Design review of the part built by this model. Coordinates are the model's own, in mm. A direction names the side the tool comes from. Coordinates: 2 decimals unless noted, no trailing zeros. Loops run counter-clockwise (first coordinate to the right, second up) from the corner with the lowest first, then second, coordinate; pieces in that order, holes last. Notation, with made-up numbers: (-17, 88.25) -> (7, 88.25) arc R25 ccw to (7, 125.25) -> close; hole circle Ø1 at (86, 33). An arc over 180 degrees is marked (long way). Answer as a JSON object with one key per item and string values.
Autodesk Inventor part; units mm, degrees
ref_plane "YZ Plane" through (0, 0, 0) normal (1, 0, 0) x (0, 1, 0)
ref_plane "XZ Plane" through (0, 0, 0) normal (0, 1, 0) x (-1, 0, 0)
ref_plane "XY Plane" through (0, 0, 0) normal (0, 0, 1) x (1, 0, 0)
sketch "TopSketch" plane through (0, 0, 0) normal (0, 1, 0) x (-1, 0, 0)
  line L0 (-39.75, -16.5) -> (39.75, -16.5)
  line L1 (39.75, -16.5) -> (39.75, 16.5)
  line L2 (39.75, 16.5) -> (-39.75, 16.5)
  line L3 (-39.75, 16.5) -> (-39.75, -16.5)
  line L4 (-39.75, -16.5) -> (39.75, 16.5) construction
  line L5 (39.75, -16.5) -> (-39.75, 16.5) construction
  point P0 (0, 0)
  dimension "EncoderSupportOutside_Length" = 33
  dimension "EncoderSupportOutside_Width" = 79.5
extrude "Top" add sketch "TopSketch" along normal blind 10
sketch "SideSketch" plane through (0, 0, 0) normal (0, -1, 0) x (1, 0, 0)
  line L0 (39.75, -16.5) -> (-39.75, -16.5)
  line L1 (39.75, 16.5) -> (39.75, -16.5)
  line L2 (-39.75, 16.5) -> (39.75, 16.5)
  line L3 (-39.75, -16.5) -> (-39.75, 16.5)
  line L4 (-29.75, 16.5) -> (-29.75, -16.5)
  line L5 (29.75, 16.5) -> (29.75, -16.5)
  line L6 (0, 0) -> (0, 21.6169) construction
  dimension "d4" = 10
extrude "Side" add sketch "SideSketch" along normal blind 51.5 contours L0 L5 L2 L1 | L0 L3 L2 L4
sketch "CableHoleSketch" plane through (0, 10, 0) normal (0, 1, 0) x (1, 0, 0)
  line L0 (-39.75, -16.5) -> (39.75, -16.5)
  line L1 (39.75, -16.5) -> (39.75, 16.5)
  line L2 (0, 0) -> (0, 14.5107) construction
  circle A0 centre (0, 18.5) radius 4.75
  dimension "d7" = 9.5
  dimension "d8" = 35
extrude "CableHole" cut sketch "CableHoleSketch" against normal up to next
sketch "InnerFasteningHoleSketch" plane through (0, 10, 0) normal (0, 1, 0) x (1, 0, 0)
  line L0 (39.75, 16.5) -> (-39.75, 16.5)
  line L1 (39.75, 16.5) -> (-39.75, 16.5)
  circle A0 centre (-24.25, 11.5) radius 2
  line L2 (0, 0) -> (39.099, 0) construction
  line L3 (0, 0) -> (0, 35.9734) construction
  circle A1 centre (-24.25, -11.5) radius 2
  circle A2 centre (24.25, 11.5) radius 2
  circle A3 centre (24.25, -11.5) radius 2
  dimension "d11" = 4
  dimension "d12" = 5
  dimension "d13" = 24.25
extrude "InnerFasteningHole" cut sketch "InnerFasteningHoleSketch" against normal up to next
sketch "OuterFasteningHoleSketch" plane through (0, 10, 0) normal (0, 1, 0) x (1, 0, 0)
  line L0 (39.75, 16.5) -> (-39.75, 16.5)
  line L1 (-39.75, 16.5) -> (-39.75, -16.5)
  line L2 (39.75, 16.5) -> (-39.75, 16.5)
  circle A0 centre (-34.75, 11.5) radius 1.75
  line L3 (0, 0) -> (36.9685, 0) construction
  line L4 (0, 0) -> (0, 24.5431) construction
  circle A1 centre (34.75, 11.5) radius 1.75
  circle A2 centre (-34.75, -11.5) radius 1.75
  circle A3 centre (34.75, -11.5) radius 1.75
  dimension "d16" = 3.5
  dimension "d17" = 5
  dimension "d18" = 5
extrude "OuterFasteningHole" cut sketch "OuterFasteningHoleSketch" against normal up to next
sketch "CoilSpringHoleSketch" plane through (0, 0, 0) normal (0, -1, 0) x (1, 0, 0)
  circle A0 centre (24.25, -11.5) radius 2
  circle A1 centre (-24.25, -11.5) radius 2
  circle A2 centre (-24.25, 11.5) radius 2
  circle A3 centre (24.25, 11.5) radius 2
  line L0 (29.75, -16.5) -> (-29.75, -16.5)
  circle A4 centre (-24.25, 11.5) radius 3
  line L1 (0, 0) -> (0, 23.1959) construction
  line L2 (0, 0) -> (47.7515, 0) construction
  circle A5 centre (24.25, 11.5) radius 3
  circle A6 centre (-24.25, -11.5) radius 3
  circle A7 centre (24.25, -11.5) radius 3
  point P0 (-4.3084, -16.5)
  dimension "d21" = 6
extrude "CoilSpringHole" cut sketch "CoilSpringHoleSketch" against normal blind 5
sketch "Sketch7" plane through (0, 0, 0) normal (0, -1, 0) x (1, 0, 0)
  circle A0 centre (-24.25, 11.5) radius 3
  arc A1 (4.3084, -16.5) -> (-4.3084, -16.5) centre (0, -18.5) ccw
  line L0 (-29.75, 16.5) -> (-29.75, -16.5)
  line L1 (-29.75, 5.5) -> (-23, 5.5)
  line L2 (-23, 5.5) -> (-23, -5.5)
  line L3 (-23, -5.5) -> (-29.75, -5.5)
  line L4 (-29.75, -5.5) -> (-29.75, 5.5)
  line L5 (0, 0) -> (50.1862, 0) construction
  line L6 (0, 0) -> (0, -18.5) construction
  line L7 (29.75, 5.5) -> (23, 5.5)
  line L8 (23, 5.5) -> (23, -5.5)
  line L9 (23, -5.5) -> (29.75, -5.5)
  line L10 (29.75, -5.5) -> (29.75, 5.5)
  circle A2 centre (-24.25, 11.5) radius 3 construction
  dimension "d25" = 3
  dimension "d26" = 23
extrude "Extrusion7" add sketch "Sketch7" along normal up to surface (51.5 mm away) contours L1 L2 L3 L0 | L10 L9 L8 L7
fillet "Fillet" radius 2 8 edges at (-29.75, -25.75, 5.5) (-23, -25.75, 5.5) (-23, -25.75, -5.5) (-29.75, -25.75, -5.5) (29.75, -25.75, 5.5) (23, -25.75, 5.5) (23, -25.75, -5.5) (29.75, -25.75, -5.5)
fillet "Fillet" radius 2 10 edges at (39.75, -20.75, -16.5) (-39.75, -20.75, -16.5) (22.0292, 10, -16.5) (0, 10, -13.75) (-22.0292, 10, -16.5) (39.75, 10, 0) (0, 10, 16.5) (-39.75, 10, 0) (-39.75, -20.75, 16.5) (39.75, -20.75, 16.5)
equation "\"EncoderSupportOutside_Length\" = EncoderSupportInside_Length"
equation "\"EncoderSupportOutside_Width\" = EncoderSupportInside_Width + 2 * EncoderSupportOutside_Thickness + 2 * EncoderSupportOutside_MecanicalSpace"
equation "\"d2\" = EncoderSupportOutside_Thickness"
equation "\"d4\" = EncoderSupportOutside_Thickness"
equation "\"d5\" = EncoderSupportInside_Height + EncoderSupport_Space"
equation "\"d7\" = Encoder_CableBase_Diameter + EncoderSupport_PlasticShrinkingMargin"
equation "\"d8\" = Encoder_CableBase_DistanceToTop + EncoderSupportInside_Front_Thickness"
equation "\"d9\" = EncoderSupportOutside_Thickness"
equation "\"d11\" = EncoderSupport_PlasticShrinkingMargin + EncoderSupport_FixingHole_Diameter + EncoderSupportOutside_MecanicalSpace"
equation "\"d12\" = EncoderSupport_FixingnHole_Margin"
equation "\"d14\" = EncoderSupportOutside_Thickness"
equation "\"d16\" = EncoderSupport_FixingHole_Diameter + EncoderSupport_PlasticShrinkingMargin"
equation "\"d17\" = EncoderSupport_FixingnHole_Margin"
equation "\"d18\" = EncoderSupport_FixingnHole_Margin"
equation "\"d19\" = EncoderSupportOutside_Thickness"
equation "\"d21\" = EncoderSupport_CoilSpringHole_Diameter"
equation "\"d25\" = EncoderSupportInside_Hollow_Margin + EncoderSupportOutside_MecanicalSpace"
equation "\"d29\" = EncoderSupport_Fillet_Size"
equation "\"EncoderSupportOutside_Thickness\" = 10"
equation "\"EncoderSupportOutside_MecanicalSpace\" = 0.5"
equation "\"EncoderSupport_Space\" = 5"
properties part number "EncoderSupportOutside" material "Polyethylene, High Density"
1) Add section C-C, the plane x = 34.75. Give the boundary of the cut face in (y, z), and give its area (3 significant figures).
Completed:
{"outline": "(-51.5, -16.5) -> (8, -16.5) arc R2 ccw to (10, -14.5) -> (10, -13.25) -> (-51.5, -13.25) -> close; (-51.5, -9.75) -> (10, -9.75) -> (10, 9.75) -> (-51.5, 9.75) -> close; (-51.5, 13.25) -> (10, 13.25) -> (10, 14.5) arc R2 ccw to (8, 16.5) -> (-51.5, 16.5) -> close", "area": "1,600 mm²"}
2) The part is to be moulded in two halves that separate along Z. For faces 4 (the cylindrical face through (-27.247, 2.465, 11.632)), 5 (the flat face through (-33, -51.5, 0)), 6 (the flat face through (26, -25, -5.5)), say which applies: pulls with the +Z half, pulls with the -Z half, needs draft (parallel to the pull), parting line crosses it, or undercut.
Completed:
{"face 4": "undercut", "face 5": "needs draft", "face 6": "pulls with the -Z half"}
3) Clearance check with flat-ended pins moving along their axes: pin 1 Ø6.5 at (x, z) = (-25.5, -12) entering from -Y; pin 2 Ø0.8 at (x, y) = (26, -14.5) entering from -Z; pin 3 Ø0.8 at (x, y) = (26, -18) entering from +Z. State where each tip first meets the part, or that it passes through.
Completed:
{"pin 1": "y = 0", "pin 2": "z = -5.5", "pin 3": "z = 5.5"}
4) For faces 1 (the flat face through (-22, 5, -12)), 2 (the cylindrical face through (23.6, -26.11, 4.93)), 3 (the flat face through (23, -25, 0)), list the 3-axis set-ups (+Z, -Z, +X, -X, +Y, -Y) from which the entire face can be reached by the end or side of a thin tool; tool diameter is ignored.
Completed:
{"face 1": "-Y", "face 2": "+Z, -Y", "face 3": "+Z, -Z, -Y"}
5) Add section D-D, the plane z = -0.5. Give the boundary of the cut face in (x, y), and give its area (3 significant figures).
Completed:
{"outline": "(-39.75, -51.5) -> (-23, -51.5) -> (-23, 0) -> (23, 0) -> (23, -51.5) -> (39.75, -51.5) -> (39.75, 8) arc R2 ccw to (37.75, 10) -> (-37.75, 10) arc R2 ccw to (-39.75, 8) -> close", "area": "2,520 mm²"}
6) Add section A-A, the plane z = 11.5. Count the separate pieces of the cut face and the enclosed holes in it, and give its area (3 significant figures).
Completed:
{"separate pieces": "5", "enclosed holes": "0", "area": "1,290 mm²"}
7) Wall thickness on probe 1 along Z at (x, y) = (-34.75, -24.5); probe 2 along Z at (x, y) = (-24.25, 3.25); probe 3 along X at (y, z) = (-27, -11.5): over which ranges is each line inside the solid? List them lowest first.
Completed:
{"probe 1": "-16.5 to -13.25, -9.75 to 9.75, 13.25 to 16.5", "probe 2": "-16.5 to -14.5, -8.5 to 8.5, 14.5 to 16.5", "probe 3": "-39.75 to -36.5, -33 to -29.75, 29.75 to 33, 36.5 to 39.75"}
